Geometry: final body of the model. Coordinates: model frame, mm. Round coordinates to 2 decimals unless told otherwise and drop trailing zeros. Loops run counter-clockwise (first coordinate to the right, second up) from the corner with the lowest first, then second, coordinate; pieces in that order, holes last. Notation, with made-up numbers: M 66.5,-30 L 118.5,-30 A18 ccw 118.5,-18 Z; hole C 61.5,54.25 d5. An arc over 180 degrees is marked long. Answer as a JSON object with one key per item and string values.
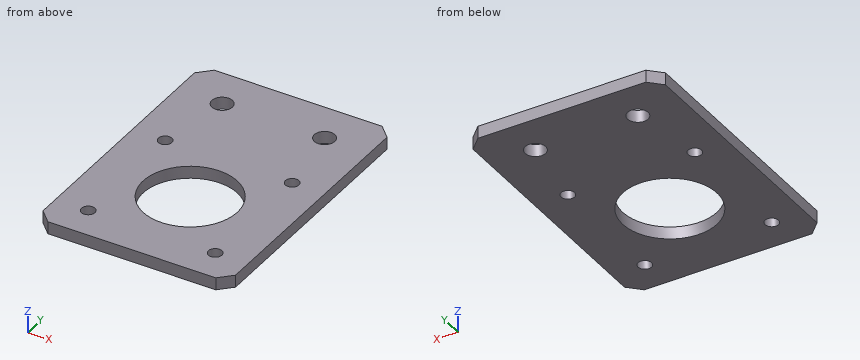
Autodesk Fusion 360 part; units mm, degrees
sketch "Skizze1" plane through (0, 0, 0) normal (0, 0, 1) x (1, 0, 0)
  circle A0 centre (0, 0) radius 11.5
  line L0 (23.5, -23.5) -> (-23.5, -23.5)
  line L1 (-23.5, -23.5) -> (-23.5, 23.5)
  line L2 (-23.5, 23.5) -> (23.5, 23.5)
  line L3 (23.5, 23.5) -> (23.5, -23.5)
  line L4 (23.5, -23.5) -> (-23.5, 23.5) construction
  line L5 (-23.5, -23.5) -> (23.5, 23.5) construction
  line L6 (21.5, -21.5) -> (-21.5, -21.5) construction
  line L7 (-21.5, -21.5) -> (-21.5, 21.5) construction
  line L8 (-21.5, 21.5) -> (21.5, 21.5) construction
  line L9 (21.5, 21.5) -> (21.5, -21.5) construction
  line L10 (21.5, -21.5) -> (-21.5, 21.5) construction
  line L11 (-21.5, -21.5) -> (21.5, 21.5) construction
  line L12 (15.5, -15.5) -> (-15.5, -15.5) construction
  line L13 (-15.5, -15.5) -> (-15.5, 15.5) construction
  line L14 (-15.5, 15.5) -> (15.5, 15.5) construction
  line L15 (15.5, 15.5) -> (15.5, -15.5) construction
  line L16 (15.5, -15.5) -> (-15.5, 15.5) construction
  line L17 (-15.5, -15.5) -> (15.5, 15.5) construction
  circle A1 centre (-15.5, 15.5) radius 1.65
  circle A2 centre (15.5, 15.5) radius 1.65
  circle A3 centre (15.5, -15.5) radius 1.65
  circle A4 centre (-15.5, -15.5) radius 1.65
  line L18 (-23.5, 23.5) -> (-23.5, 43.5)
  line L19 (-23.5, 43.5) -> (23.5, 43.5)
  line L20 (23.5, 43.5) -> (23.5, 23.5)
  line L21 (-23.5, 33.5) -> (23.5, 33.5) construction
  circle A5 centre (-12.5, 33.5) radius 2.5
  circle A6 centre (12.5, 33.5) radius 2.5
  line L22 (0, 1.75) -> (0, 22.5)
  dimension "d120" = 43
  dimension "d121" = 23
  dimension "d122" = 2
  dimension "d123" = 31
  dimension "d124" = 3.3
  dimension "d125" = 2
  dimension "d126" = 20
  dimension "d127" = 5
  dimension "d128" = 25
extrude "Extrusion1" add sketch "Skizze1" along normal blind 3
chamfer "Fase1" distance 3 angle 45 4 edges at (-23.5, -23.5, 1.5) (23.5, -23.5, 1.5) (23.5, 43.5, 1.5) (-23.5, 43.5, 1.5)
equation "frame_outer_x = 400 mm"
equation "frame_outer_y = 400 mm"
equation "frame_outer_z = 600 mm"
equation "M3_hole_dia = 3.5 mm"
equation "M4_hole_dia = 4.5 mm"
equation "M5_hole_dia = 5.2 mm"
equation "M6_hole_dia = 6.2 mm"
equation "M3_hole_dia_thread = 2.6 mm"
equation "M4_hole_dia_thread = 3.4 mm"
equation "M5_hole_dia_thread = 4.3 mm"
equation "M6_hole_dia_thread = 5.2 mm"
equation "M3_head_dia = 6 mm"
equation "M4_head_dia = 7 mm"
equation "M5_head_dia = 9 mm"
equation "M6_head_dia = 11 mm"
equation "M3_head_height = 3 mm"
equation "M4_head_height = 4 mm"
equation "M5_head_height = 5 mm"
equation "M6_head_height = 6 mm"
equation "nema_17_outer_XY = 43 mm"
equation "nema_17_outer_z = 40 mm"
equation "nema_17_screw_distance = 31 mm"
equation "nema_17_center_ring_dia = 23 mm"
equation "nema_17_center_ring_height = 2 mm"
equation "nema_17_shaft_length = 24 mm"
equation "nema_17_shaft_dia = 5 mm"
equation "lm8uu_outer_dia = 15 mm"
equation "lm8uu_length = 24 mm"
equation "lm8uu_nut_distance_cc = 16.4 mm"
equation "scs8uu_lenght = 30 mm"
equation "scs8uu_width = 34.4 mm"
equation "scs8uu_screw_distance_cc_1 = 18 mm"
equation "scs8uu_screw_distance_cc_2 = 24 mm"
equation "scs8uu_base_road_cc = 11 mm"
equation "scs8uu_screw_hole_dia = 4 mm"
equation "lmk8luu_length = 45 mm"
equation "lmk8luu_head_xy = 25 mm"
equation "lmk8luu_body_dia = 15 mm"
equation "lmk8luu_circle_holes_dia = 24 mm"
equation "lmk8luu_screw_hole_dia = 3 mm"
equation "kp08_screw_distance_cc = 42 mm"
equation "kp08_base_road_cc = 15 mm"
equation "kp08_screw_hole_dia = 4 mm"
equation "sk8_screw_distance_cc = 32 mm"
equation "sk8_base_road_cc = 20 mm"
equation "sk8_screw_hole_dia = 5 mm"
equation "trapezoidal_screw_z_length = 300 mm"
equation "coupler_5x8_length = 25 mm"
equation "coupler_5x8_outer_dia = 19 mm"
equation "t8_nut_outer_dia_1 = 22 mm"
equation "t8_nut_outer_dia_2 = 10.2 mm"
equation "t8_nut_screw_hole_dia = 3 mm"
equation "t8_nut_screw_circle_holes_dia = 16 mm"
equation "heatbed_outer_x = 220 mm"
equation "heatbed_outer_y = 220 mm"
equation "heatbed_x_srew_cc = 210 mm"
equation "heatbed_y_srew_cc = 210 mm"
equation "x_rods_distance_cc = 40 mm"
equation "y_rods_distance_cc = 140 mm"
equation "z_rods_distance_cc = 300 mm"
equation "steel_rods_dia = 8.2 mm"
equation "x_profile_distance_cc = 60 mm"
equation "y_profile_distance_cc = 160 mm"
equation "z_profile_distance_cc = 300 mm"
equation "x_profile_length = 300 mm"
equation "y_profile_length = 300 mm"
equation "z_profile_length = 300 mm"
equation "y_profile_xy = 20 mm"
equation "z_profil_x = 20 mm"
equation "z_profil_y = 40 mm"
equation "profil_nut_width = 6 mm"
equation "profil_nut_depth = 5 mm"
equation "pulley_gt2_20t_outer_dia = 16 mm"
equation "pulley_gt2_20t_inner_dia = 12.2 mm"
equation "pulley_gt2_16t_outer_dia = 13.8 mm"
equation "pulley_gt2_16t_inner_dia = 9.4 mm"
equation "e3d_heigh_all = 62.3 mm"
equation "e3d_mounting_dia_inner = 12 mm"
equation "e3d_mounting_dia_outer = 16 mm"
equation "e3d_mounting_height = 6 mm"
equation "e3d_upper_mount_height = 3.7 mm"
equation "e3d_distance_nozzle_mounting_center = e3d_heigh_all - ( e3d_mounting_height / 2 ) - e3d_upper_mount_height"
equation "f624_zz_outer_dia = 15 mm"
equation "f624_zz_inner_dia = 13 mm"
equation "f624_zz_hole_dia = 4 mm"
equation "f623_zz_outer_dia = 11.5 mm"
equation "f623_zz_inner_dia = 10 mm"
equation "f623_zz_hole_dia = 3 mm"
equation "fan_30x30_xy_outside = 30 mm"
equation "fan_30x30_xy_screw_distance = 24 mm"
equation "fan_30x30_fan_opening_dia = 28 mm"
equation "fan_40x40_xy_outside = 40 mm"
equation "fan_40x40_xy_screw_distance = 32 mm"
equation "fan_40x40_fan_opening_dia = 38 mm"
equation "fan_50x50_xy_outside = 50 mm"
equation "fan_50x50_xy_screw_distance = 40 mm"
equation "fan_50x50_fan_opening_dia = 47 mm"
equation "fan_60x60_xy_outside = 60 mm"
equation "fan_60x60_xy_screw_distance = 51 mm"
equation "fan_60x60_fan_opening_dia = 57 mm"
equation "fan_12x120_xy_outside = 120 mm"
equation "fan_12x120_xy_screw_distance = 105 mm"
equation "fan_12x120_fan_opening_dia = 116 mm"
equation "d120 = nema_17_outer_XY"
equation "d121 = nema_17_center_ring_dia"
equation "d123 = nema_17_screw_distance"
1) Line query: probe 1 along Y at (x, z) = (-15.5, 2); probe 2 along Y at (x, z) = (-12.5, 1.45); probe 3 along Y at (x, z) = (0.5, 1.3). Output: solid intervals per line, ascending.
Geometry results:
{"probe 1": "-23.5 to -17.15, -13.85 to 13.85, 17.15 to 43.5", "probe 2": "-23.5 to 31, 36 to 43.5", "probe 3": "-23.5 to -11.49, 11.49 to 43.5"}
2) Cut plane C-C on y = 0. Return the cut outline in (x, z), and give its area (3 significant figures).
Geometry results:
{"outline": "M -23.5,0 L -11.5,0 L -11.5,3 L -23.5,3 Z; M 11.5,0 L 23.5,0 L 23.5,3 L 11.5,3 Z", "area": "72.0 mm2"}
3) Cut plane D-D on z = 2.5. Return the cut outline in (x, y).
Geometry results:
{"outline": "M -23.5,-20.5 L -20.5,-23.5 L 20.5,-23.5 L 23.5,-20.5 L 23.5,40.5 L 20.5,43.5 L -20.5,43.5 L -23.5,40.5 Z; hole C -15.5,-15.5 d3.3; hole C -15.5,15.5 d3.3; hole C -12.5,33.5 d5; hole C 0,0 d23; hole C 12.5,33.5 d5; hole C 15.5,-15.5 d3.3; hole C 15.5,15.5 d3.3"}
4) Cut plane A-A on y = 33.5. Return the cut outline in (x, z).
Geometry results:
{"outline": "M -23.5,0 L -15,0 L -15,3 L -23.5,3 Z; M -10,0 L 10,0 L 10,3 L -10,3 Z; M 15,0 L 23.5,0 L 23.5,3 L 15,3 Z"}
5) Cut plane B-B on x = 12.5. Return the cut outline in (y, z).
Geometry results:
{"outline": "M -23.5,0 L 31,0 L 31,3 L -23.5,3 Z; M 36,0 L 43.5,0 L 43.5,3 L 36,3 Z"}
